Verification items for the finished model (mm, model axes). A direction names the side the tool comes from. Coordinates: 2 decimals unless noted, no trailing zeros. Loops run counter-clockwise (first coordinate to the right, second up) from the corner with the lowest first, then second, coordinate; pieces in that order, holes last. Notation, with made-up numbers: (82, 38.5) -> (137, 38.5) arc R34 cw to (137, 68.5) -> close; hole circle Ø10 at (35, -34). An arc over 180 degrees is marked (long way). Write item = value, one per line.
```python
from build123d import *

# Parameters (mm, degrees)
SKETCH1_W           = 31.75
SKETCH1_H           = 31.75
BOSS_EXTRUDE1_DEPTH = 19.05
SKETCH2_R           = 9.525
SKETCH2_R_2         = 3.175
BOSS_EXTRUDE2_DEPTH = 19.05
FILLET1_R           = 6.35


with BuildPart() as part:
    # Sketch1 → Boss-Extrude1 (new body)
    with BuildSketch(Plane(origin=(0, 0, 0), x_dir=(0, 0, -1), z_dir=(1, 0, 0))):
        Rectangle(SKETCH1_W, SKETCH1_H)
    extrude(amount=BOSS_EXTRUDE1_DEPTH)

    # Sketch2 → Boss-Extrude2 (add)
    with BuildSketch(Plane(origin=(19.05, 0, 0), x_dir=(0, 0, -1), z_dir=(1, 0, 0))):
        with Locations(Location((0, 0, 0), (0, 0, 180))):
            Circle(SKETCH2_R)
        with Locations(Location((0, 0, 0), (0, 0, 180))):
            Circle(SKETCH2_R_2, mode=Mode.SUBTRACT)
    extrude(amount=BOSS_EXTRUDE2_DEPTH)

    # Fillet1
    fillet1_edges = [part.edges().sort_by_distance(p)[0] for p in [
        (9.525, -15.875, -15.875),
        (9.525, -15.875, 15.875),
        (9.525, 15.875, 15.875),
        (9.525, 15.875, -15.875),
    ]]
    fillet(fillet1_edges, radius=FILLET1_R)


solid = part.part
```
1) Material ranges on line 1 (Y direction, x = 33, z = 0) (3 decimals); line 2 (X direction, y = -5.5, z = 8); line 3 (Z direction, x = 25.5, y = -3.5), recorded low to high.
Ans:
line_1 = -9.525 to -3.175, 3.175 to 9.525
line_2 = 0 to 19.05
line_3 = -8.86 to 8.86
2) Depth check by flat-ended pin: pin 1 Ø1.5 at (y, z) = (1.5, -1) entering from +X; pin 2 Ø12 at (x, y) = (20.5, 7.5) entering from -Z (3 decimals); pin 3 Ø10 at (x, z) = (31.5, 10) entering from +Y; pin 4 Ø6 at (x, y) = (24, -9.5) entering from -Z. Enter the tip coordinate at first touch or a pass-through.
Ans:
pin_1 = 19.05
pin_2 = -15.875
pin_3 = 8.11
pin_4 = -6.96
3) Sectioned sample at D-D, the plane x = 26.5. Record the cut outline in (y, z) (3 decimals), plus the area to 3 significant figures.
Ans:
outline = circle Ø19.05 at (0, 0); hole circle Ø6.35 at (0, 0)
area = 253 mm2
4) Release check for a two-part mould opening along Z. For faces 3 (the face through (9, 0, -15.875)), 4 (the face through (28.4, 2.8, 1.5)), 5 (the face through (9, 15.875, 0)), 6 (the face through (19.05, 0, 0)) record: pulls with the +Z half, pulls with the -Z half, needs draft (parallel to the pull), parting line crosses it, or undercut.
Ans:
face_3 = pulls with the -Z half
face_4 = undercut
face_5 = needs draft
face_6 = undercut
5) Sectioned sample at A-A, the plane x = 15. Record the cut outline in (y, z) (3 decimals), plus the area to 3 significant figures.
Ans:
outline = (-15.875, -9.525) arc R6.35 ccw to (-9.525, -15.875) -> (9.525, -15.875) arc R6.35 ccw to (15.875, -9.525) -> (15.875, 9.525) arc R6.35 ccw to (9.525, 15.875) -> (-9.525, 15.875) arc R6.35 ccw to (-15.875, 9.525) -> close
area = 973 mm2
6) Tool access check on faces 1 (the face through (28.44, 9.3, -2.06)), 2 (the face through (9, -15.875, 0)). Record the directions out of +Z, -Z, +X, -X, +Y, -Y that give a thin tool (end or side, any length) a straight path to the whole face; none if there is none.
Ans:
face_1 = +X
face_2 = +Z, -Z, +X, -X, -Y
7) Sectioned sample at B-B, the plane z = 0. Record the cut outline in (x, y) (3 decimals).
Ans:
outline = (0, -15.875) -> (19.05, -15.875) -> (19.05, -9.525) -> (38.1, -9.525) -> (38.1, -3.175) -> (19.05, -3.175) -> (19.05, 3.175) -> (38.1, 3.175) -> (38.1, 9.525) -> (19.05, 9.525) -> (19.05, 15.875) -> (0, 15.875) -> close
